Input: part model. Units: mm. Frame: model coordinates. Face numbers are marked on the shaded views. Give positions to 0.01 mm unless a question says otherwise; leave off trailing zeros. Write each loop counter-clockwise with the first axis right and the second up, starting at its lowest first coordinate (ties: lowest second). Pieces come first, ordered by that corner, then holes. Notation, with made-up numbers: (32, 4) - (88, 4) arc R34 ccw to (88, 35) - close; hole circle Ø6 at (-15, 53.25). An arc over 180 degrees is marked (long way). Answer as a JSON object with one key per item and string values. Group by question number.
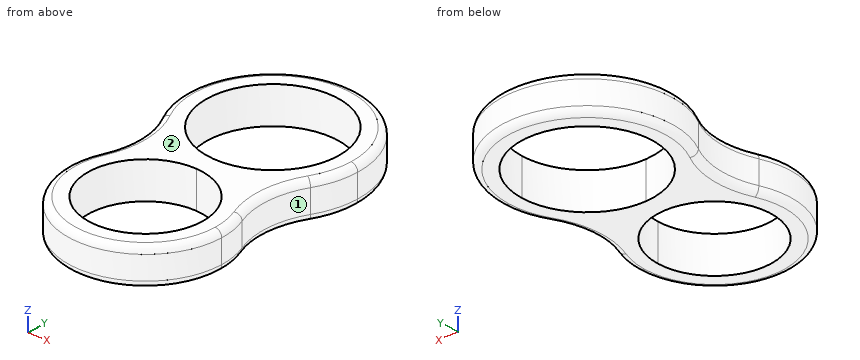
from build123d import *

# Parameters (mm, degrees)
F1_DEPTH = 6.985
F2_R     = 1.27


with BuildPart() as f1:
    # F0 (on Top) → F1 (new body)
    with BuildSketch(Plane.XY):
        with BuildLine():
            ThreePointArc((-13.7046532603, 5.6428322521), (-11.1770065001, 9.7331188478), (-7.4729632817, 12.7989802953))
            ThreePointArc((-7.4729632817, 12.7989802953), (-11.487981867, 15.6631441995), (-14.4778651692, 19.5854403319))
            ThreePointArc((-14.4778651692, 19.5854403319), (-12.5103993427, 12.7018056629), (-13.7046532603, 5.6428322521))
        make_face()
        with BuildLine():
            ThreePointArc((14.4771044871, 19.5840526618), (11.4874135696, 15.6625936504), (7.4729632817, 12.7989802953))
            ThreePointArc((7.4729632817, 12.7989802953), (11.1765146122, 9.7336836774), (13.7040828571, 5.644217382))
            ThreePointArc((13.7040828571, 5.644217382), (12.5096874073, 12.7018028253), (14.4771044871, 19.5840526618))
        make_face()
        with BuildLine():
            ThreePointArc((7.4729632817, 12.7989802953), (3.8419529979, 11.4641413868), (0, 11.0109))
            ThreePointArc((0, 11.0109), (-3.8419529979, 11.4641413868), (-7.4729632817, 12.7989802953))
            ThreePointArc((-7.4729632817, 12.7989802953), (-11.1770065001, 9.7331188478), (-13.7046532603, 5.6428322521))
            ThreePointArc((-13.7046532603, 5.6428322521), (-2.8760894722, -14.5391604351), (14.8209, 0))
            ThreePointArc((14.8209, 0), (14.5390150703, 2.8768242207), (13.7040828571, 5.644217382))
            ThreePointArc((13.7040828571, 5.644217382), (11.1765146122, 9.7336836774), (7.4729632817, 12.7989802953))
        make_face()
        with BuildLine():
            ThreePointArc((0, 11.0109), (7.785882057, 7.785882057), (11.0109, 0))
            ThreePointArc((11.0109, 0), (-7.785882057, -7.785882057), (0, 11.0109))
        make_face(mode=Mode.SUBTRACT)
        with BuildLine():
            ThreePointArc((-7.4729632817, 12.7989802953), (-3.8708312936, 14.3064929982), (-7.5e-09, 14.8209))
            ThreePointArc((-7.5e-09, 14.8209), (3.8708312864, 14.3064930001), (7.4729632817, 12.7989802953))
            ThreePointArc((7.4729632817, 12.7989802953), (11.4874135696, 15.6625936504), (14.4771044871, 19.5840526618))
            ThreePointArc((14.4771044871, 19.5840526618), (15.9937033717, 23.4243706813), (16.51, 27.5209))
            ThreePointArc((16.51, 27.5209), (-4.095762814, 43.5147996799), (-14.4778651692, 19.5854403319))
            ThreePointArc((-14.4778651692, 19.5854403319), (-11.487981867, 15.6631441995), (-7.4729632817, 12.7989802953))
        make_face()
        with BuildLine():
            ThreePointArc((12.7, 27.5209), (8.9802561184, 18.5406438763), (-7.5e-09, 14.8209))
            ThreePointArc((-7.5e-09, 14.8209), (-8.9802561184, 36.5011561237), (12.7, 27.5209))
        make_face(mode=Mode.SUBTRACT)
        with BuildLine():
            Line((0, 14.8209), (0, 11.0109))
            ThreePointArc((0, 11.0109), (3.8419529979, 11.4641413868), (7.4729632817, 12.7989802953))
            ThreePointArc((7.4729632817, 12.7989802953), (3.8708312864, 14.3064930001), (-7.5e-09, 14.8209))
        make_face()
        with BuildLine():
            ThreePointArc((-7.4729632817, 12.7989802953), (-3.8419529979, 11.4641413868), (0, 11.0109))
            Line((0, 11.0109), (0, 14.8209))
            ThreePointArc((-7.5e-09, 14.8209), (-3.8708312936, 14.3064929982), (-7.4729632817, 12.7989802953))
        make_face()
    extrude(amount=F1_DEPTH)

    # F2
    f2_edges = [f1.edges().sort_by_distance(p)[0] for p in [
        (0.000791, 44.0309, 6.985),
        (0.000791, 44.0309, 0),
    ]]
    fillet(f2_edges, radius=F2_R)


solid = f1.part
1) Line query: line 1 along Y through (x, z) = (0, 2.25); line 2 along Y through (x, z) = (4, 3); line 3 along X through (y, z) = (0, 3.5). Output: solid intervals per line, ascending. Write a range as from..to.
2) Mould query, pull axis Y, two halves, no side actions, for the marked faces 1 and 2. Classes: +Y half, -Y half, draft (parallel to the pull), parting line (faces both ways), or undercut.
3) Cut plane A-A on z = 2. Return the cut outline in (x, y), and give its area (3 significant figures).
4) Pin query (flat end, axial travel): P1, Ø4, axis at y = 8.5, z = 5, coming from the -X side; P2, Ø3, axis at y = -5, z = 6, coming from the +X side; P3, Ø1.5, axis at x = -1, z = 0.5, coming from the +Y side. Return the tip coordinate at first contact, or that it passes through.
5) Cut plane B-B on x = -4.5. Count the separate pieces of the cut face and the enclosed holes in it, and give its area (3 significant figures).
Filled in:
{
 "1": {"line 1": "y = -14.82..-11.01, 11.01..14.82, 40.22..44.03", "line 2": "y = -14.27..-10.26, 10.26..15.47, 39.57..43.54", "line 3": "x = -14.82..-11.01, 11.01..14.82"},
 "2": {"face 1": "undercut", "face 2": "draft"},
 "3": {"outline": "(-14.48, 19.59) arc R16.19 cw to (-13.7, 5.64) arc R14.82 ccw (long way) to (13.7, 5.64) arc R16.18 cw to (14.48, 19.58) arc R16.51 ccw (long way) to start; hole circle Ø25.4 at (0, 27.52); hole circle Ø22.02 at (0, 0)", "area": "663 mm²"},
 "4": {"P1": "stops at x = -13.38", "P2": "stops at x = 14.4", "P3": "stops at y = 44.01"},
 "5": {"separate pieces": "3", "enclosed holes": "0", "area": "94.1 mm²"}
}
